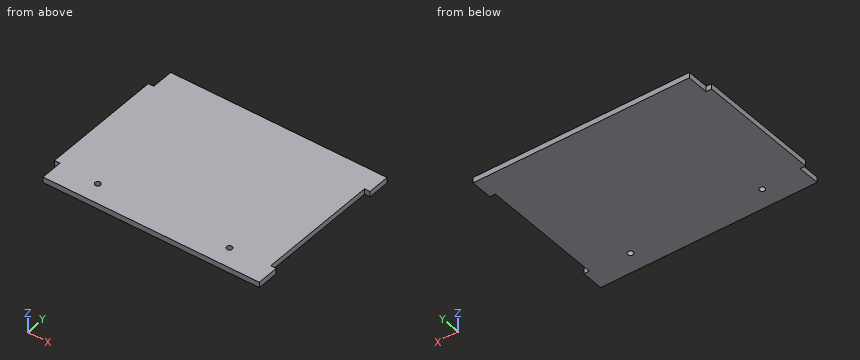
```python
from build123d import *

# Parameters (mm, degrees)
SKETCH_R  = 2.5
PAD_DEPTH = 2.5


with BuildPart() as part:
    # Sketch → Pad (new body, symmetric)
    with BuildSketch(Plane.XY):
        Polygon((98.5, 55.5), (98.5, 75.5), (-98.5, 75.5), (-98.5, 55.5), (-103.5, 55.5), (-103.5, -55.5), (-98.5, -55.5), (-98.5, -75.5), (98.5, -75.5), (98.5, -55.5), (93.5, -55.5), (93.5, 55.5), align=None)
        with Locations((57.5, -57.5)):
            Circle(SKETCH_R, mode=Mode.SUBTRACT)
        with Locations((-62.5, -57.5)):
            Circle(SKETCH_R, mode=Mode.SUBTRACT)
    extrude(amount=PAD_DEPTH, both=True)


solid = part.part
```
CAD build for the part. Positions are in the model's coordinates, mm. Round coordinates to 2 decimals unless told otherwise and drop trailing zeros. Write each loop counter-clockwise with the first axis right and the second up, starting at its lowest first coordinate (ties: lowest second). Pieces come first, ordered by that corner, then holes.
Item 1: Band-saw the part on B-B on z = -0.7. Write the cut outline in (x, y), then the cut area to 3 significant figures.
Filled in:
outline: (-103.5, -55.5) - (-98.5, -55.5) - (-98.5, -75.5) - (98.5, -75.5) - (98.5, -55.5) - (93.5, -55.5) - (93.5, 55.5) - (98.5, 55.5) - (98.5, 75.5) - (-98.5, 75.5) - (-98.5, 55.5) - (-103.5, 55.5) - close; hole circle Ø5 at (-62.5, -57.5); hole circle Ø5 at (57.5, -57.5)
area: 29,700 mm2
Item 2: Drill centre lines: L1, parallel to X at y = 37.5, z = 0.8; L2, parallel to Y at x = 57.5, z = 1.35; L3, parallel to X at y = 65, z = 0. Where is each one in solid material? Low to high.
Filled in:
L1: x = -103.5 to 93.5
L2: y = -75.5 to -60, -55 to 75.5
L3: x = -98.5 to 98.5
Item 3: Drop flat-ended pins along their axis: pin 1 Ø2.5 at (y, z) = (-64.5, 0.5) entering from -X; pin 2 Ø1.5 at (y, z) = (-14.5, -1) entering from +X. Give the stop position or say it passes through.
Filled in:
pin 1: stops at x = -98.5
pin 2: stops at x = 93.5
Item 4: Band-saw the part on C-C on y = 31.5. Write the cut outline in (x, z).
Filled in:
outline: (-103.5, -2.5) - (93.5, -2.5) - (93.5, 2.5) - (-103.5, 2.5) - close
Item 5: Band-saw the part on A-A on x = 57.5. Write the cut outline in (y, z), then the cut area to 3 significant figures.
Filled in:
outline: (-75.5, -2.5) - (-60, -2.5) - (-60, 2.5) - (-75.5, 2.5) - close; (-55, -2.5) - (75.5, -2.5) - (75.5, 2.5) - (-55, 2.5) - close
area: 730 mm2
